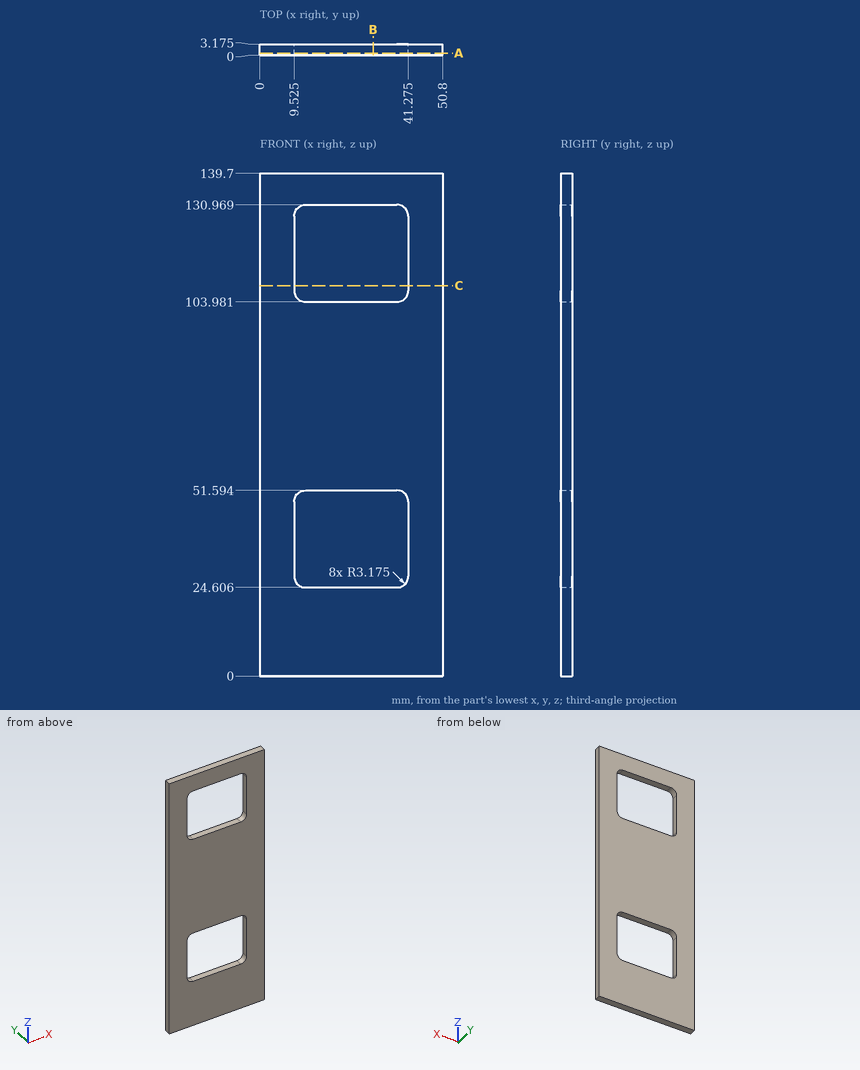
Verification items for this drawing (mm, ordinates from the low corner). Round coordinates to 2 decimals unless told otherwise and drop trailing zeros. Order: outer loops, then holes, each group sorted by start corner. A loop starts at its lowest first (then second) coordinate and runs counter-clockwise, first axis right, second up. Notation, with made-up numbers: M 13.5,47.5 L 25.5,47.5 A26 ccw 25.5,72.5 Z; hole C 18,43.5 d3. An arc over 180 degrees is marked long. Answer in a Markdown table with one row per item. Add a question column.
Item 1: Material ranges on L1, parallel to Z at x = 38, y = 0.8; L2, parallel to X at y = 0.75, z = 119 (1 decimal); L3, parallel to Z at x = 39.5, y = 1.4, recorded low to high. Write a range as [from, to].
Item 2: Sectioned sample at B-B, the plane x = 31.5. Enter the section's corners in (y, z) (1 decimal).
Item 3: Sectioned sample at A-A, the plane y = 0.65. State how many separate pieces and enclosed holes the cut face has, plus the area to 3 significant figures.
Item 4: Sectioned sample at C-C, the plane z = 108.5. Enter the section's corners in (x, y) (1 decimal), plus the area to 3 significant figures.
Filled in:
| question | item | result |
|---|---|---|
| 1 | L1 | z = [0, 24.61], [51.59, 103.98], [130.97, 139.7] |
| 1 | L2 | x = [0, 9.5], [41.3, 50.8] |
| 1 | L3 | z = [0, 24.93], [51.27, 104.31], [130.64, 139.7] |
| 2 | outline | M 0,0 L 3.2,0 L 3.2,24.6 L 0,24.6 Z; M 0,51.6 L 3.2,51.6 L 3.2,104 L 0,104 Z; M 0,131 L 3.2,131 L 3.2,139.7 L 0,139.7 Z |
| 3 | separate pieces | 1 |
| 3 | enclosed holes | 2 |
| 3 | area | 5,400 mm² |
| 4 | outline | M 0,0 L 9.5,0 L 9.5,3.2 L 0,3.2 Z; M 41.3,0 L 50.8,0 L 50.8,3.2 L 41.3,3.2 Z |
| 4 | area | 60.5 mm² |
